from build123d import *

# Parameters (mm, degrees)
BOSS_EXTRUDE1_DEPTH = 66.99
SKETCH2_R           = 5.35
CUT_EXTRUDE1_DEPTH  = 98.087126335
CUT_EXTRUDE2_DEPTH  = 92.814541877


with BuildPart() as part:
    # Sketch1 → Boss-Extrude1 (new body)
    with BuildSketch(Plane(origin=(0, 0, 0), x_dir=(1, 0, 0), z_dir=(0, 1, 0))):
        Polygon((-18.5, 1.5), (-18.5, 61.5), (-15.5, 61.5), (-15.5, 1.5), (18.5, 1.5), (18.5, -1.5), (-18.5, -1.5), align=None)
    extrude(amount=BOSS_EXTRUDE1_DEPTH)

    # Sketch2 → Cut-Extrude1 (cut, through all)
    with BuildSketch(Plane(origin=(-15.5, 0, 0), x_dir=(0, 0, -1), z_dir=(1, 0, 0))):
        with Locations((16.5, 15)):
            Circle(SKETCH2_R)
        with Locations((46.5, 51.988385001)):
            Circle(SKETCH2_R)
    extrude(amount=-CUT_EXTRUDE1_DEPTH, mode=Mode.SUBTRACT)

    # Sketch3 → Cut-Extrude2 (cut, through all)
    with BuildSketch(Plane(origin=(0, 0, -1.5), x_dir=(-1, 0, 0), z_dir=(0, 0, -1))):
        with BuildLine():
            Line((-5.25, 10), (2.25, 10))
            ThreePointArc((2.25, 10), (4.75, 7.5), (2.25, 5))
            Line((2.25, 5), (-5.25, 5))
            ThreePointArc((-5.25, 5), (-7.75, 7.5), (-5.25, 10))
        make_face()
        with BuildLine():
            Line((-5.25, 56.99), (2.25, 56.99))
            ThreePointArc((2.25, 56.99), (4.75, 59.49), (2.25, 61.99))
            Line((2.25, 61.99), (-5.25, 61.99))
            ThreePointArc((-5.25, 61.99), (-7.75, 59.49), (-5.25, 56.99))
        make_face()
    extrude(amount=-CUT_EXTRUDE2_DEPTH, mode=Mode.SUBTRACT)


solid = part.part
The model under review builds one solid part; all positions refer to its coordinate system, in mm. A direction names the side the tool comes from. Coordinates: 2 decimals unless noted, no trailing zeros. Loops run counter-clockwise (first coordinate to the right, second up) from the corner with the lowest first, then second, coordinate; pieces in that order, holes last. Notation, with made-up numbers: (-17, 69.5) -> (20, 69.5) arc R27 ccw to (20, 103.5) -> close; hole circle Ø3 at (-23, -16). An arc over 180 degrees is marked (long way). Use a Markdown table: item, result. Add a question column.
1. Clearance check with flat-ended pins moving along their axes: pin 1 Ø1.5 at (y, z) = (10.5, -54.5) entering from +X; pin 2 Ø3 at (x, y) = (13.5, 25) entering from -Z. State where each tip first meets the part, or that it passes through.
2. Add section B-B on x = 1. Write out the cut boundary in (y, z), plus the area to 3 significant figures.
3. Add section A-A on z = -46.5. Write out the cut boundary in (x, y).
4. Draft analysis for pull direction Y (two halves, no side actions). For faces 1 (the face through (0, 33, 1.5)), 2 (the face through (-16.979, 47.242, -48.969)), 3 (the face through (-16, 0, -21)), state which applies: pulls with the +Y half, pulls with the -Y half, needs draft (parallel to the pull), parting line crosses it, or undercut.
5. Machinability: for faces 4 (the face through (-4.75, 7.55, -0.02)), 5 (the face through (-16, 66.99, -21)), 6 (the face through (1, 33, -1.5)), which of the approach directions +Z, -Z, +X, -X, +Y, -Y give a long, thin tool a straight path to every point of the face, cutting with its end or side? Answer none if there is none.
6. Add section C-C on y = 59.49. Write out the cut boundary in (x, z).
7. To check wall thickness, follow line 1 (Y direction, x = -17.6, z = -46.5); line 2 (Y direction, x = -17.45, z = -16.5); line 3 (Z direction, x = -14, y = 54). State the ranges of each line that lie inside material, in increasing order.
8. Add section D-D on y = 15. Write out the cut boundary in (x, z).
Returned:
| question | item | result |
|---|---|---|
| 1 | pin 1 | stops at x = -15.5 |
| 1 | pin 2 | stops at z = -1.5 |
| 2 | outline | (0, -1.5) -> (5, -1.5) -> (5, 1.5) -> (0, 1.5) -> close; (10, -1.5) -> (56.99, -1.5) -> (56.99, 1.5) -> (10, 1.5) -> close; (61.99, -1.5) -> (66.99, -1.5) -> (66.99, 1.5) -> (61.99, 1.5) -> close |
| 2 | area | 171 mm² |
| 3 | outline | (-18.5, 0) -> (-15.5, 0) -> (-15.5, 46.64) -> (-18.5, 46.64) -> close; (-18.5, 57.34) -> (-15.5, 57.34) -> (-15.5, 66.99) -> (-18.5, 66.99) -> close |
| 4 | face 1 | needs draft |
| 4 | face 2 | undercut |
| 4 | face 3 | pulls with the -Y half |
| 5 | face 4 | +Z, -Z |
| 5 | face 5 | +Z, -Z, +X, -X, +Y |
| 5 | face 6 | -Z, +X, +Y, -Y |
| 6 | outline | (-18.5, -61.5) -> (-15.5, -61.5) -> (-15.5, -1.5) -> (-4.75, -1.5) -> (-4.75, 1.5) -> (-18.5, 1.5) -> close; (7.75, -1.5) -> (18.5, -1.5) -> (18.5, 1.5) -> (7.75, 1.5) -> close |
| 7 | line 1 | y = 0 to 46.64, 57.34 to 66.99 |
| 7 | line 2 | y = 0 to 9.65, 20.35 to 66.99 |
| 7 | line 3 | z = -1.5 to 1.5 |
| 8 | outline | (-18.5, -61.5) -> (-15.5, -61.5) -> (-15.5, -21.85) -> (-18.5, -21.85) -> close; (-18.5, -11.15) -> (-15.5, -11.15) -> (-15.5, -1.5) -> (18.5, -1.5) -> (18.5, 1.5) -> (-18.5, 1.5) -> close |
